Could you check a few things on this model? Use its own coordinates, in mm. Face numbers are marked on the shaded views. A direction names the side the tool comes from. Give positions to 0.01 mm unless a question says otherwise; leave off trailing zeros. Loops run counter-clockwise (first coordinate to the right, second up) from the corner with the lowest first, then second, coordinate; pieces in that order, holes last. Notation, with made-up numbers: (77.5, 75) - (133.5, 75) arc R16 cw to (133.5, 87) - close; hole circle Ø5 at (-39.5, 11.5). An arc over 180 degrees is marked (long way). Write each question's results on one line, items separated by ' | '. Start each with the question number.
1) On a 3-axis mill with a long thin cutter (end or side, diameter ignored), from which of +Z, -Z, +X, -X, +Y, -Y can I reach the whole of each face in a straight line? I mean the marked faces 1 and 2. Say none if no direction works.
2) I want a section at C-C, the plane y = -28.5. Write out the boundary of the cut face in (x, z), and give its area (3 significant figures).
3) I want a section at D-D, the plane x = 10. Write out the boundary of the cut face in (y, z).
4) If I drill on probe 1 along X at (y, z) = (-1.2, -15); probe 2 along Z at (x, y) = (-21, -31), over which ranges is the centre line in solid material (lowest first)? Write a range as [from, to].
5) I want a section at A-A, the plane z = -15. Write out the boundary of the cut face in (x, y), and give its area (3 significant figures).
6) I want a section at B-B, the plane x = 0. Write out the boundary of the cut face in (y, z).
7) I'm going to push flat-ended pins straight in: pin 1 (5 mm diameter, centred on x = -9.9, y = -15.2, fed in from +Z); pin 2 (12 mm diameter, centred on x = 5, z = -18, fed in from -Y); pin 3 (5 mm diameter, centred on x = 9.9, y = -15.2, fed in from -Z). Where does each tip first touch, or does it pass through?
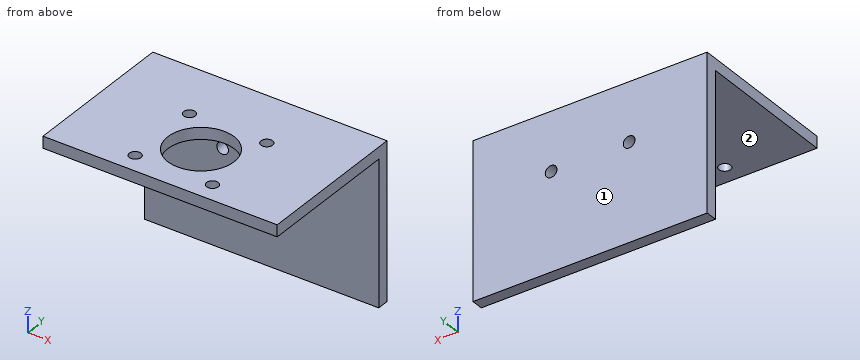
from build123d import *

# Parameters (mm, degrees)
BOSS_EXTRUDE1_DEPTH      = 30
BOSS_EXTRUDE1_DEPTH_BACK = 30
SKETCH2_R                = 1.5
SKETCH2_R_2              = 8.5
CUT_EXTRUDE1_DEPTH       = 30
SKETCH3_R                = 1.5
CUT_EXTRUDE2_DEPTH       = 30


with BuildPart() as part:
    # Sketch1 → Boss-Extrude1 (new, two sides: drawn at the far end of the back side and taken through both)
    with BuildSketch(Plane(origin=(0, 0, 0), x_dir=(0, 0, -1), z_dir=(1, 0, 0)).offset(-BOSS_EXTRUDE1_DEPTH_BACK)):
        Polygon((0, 0), (40, 0), (40, -3), (3, -3), (3, -40), (0, -40), align=None)
    extrude(amount=BOSS_EXTRUDE1_DEPTH + BOSS_EXTRUDE1_DEPTH_BACK)

    # Sketch2 → Cut-Extrude1 (cut)
    with BuildSketch(Plane.XY):
        with Locations((-9.8995, -15.201)):
            Circle(SKETCH2_R)
        with Locations((9.8995, -15.201)):
            Circle(SKETCH2_R)
        with Locations((-9.8995, -35)):
            Circle(SKETCH2_R)
        with Locations((9.8995, -35)):
            Circle(SKETCH2_R)
        with Locations((0, -25.101)):
            Circle(SKETCH2_R_2)
    extrude(amount=-CUT_EXTRUDE1_DEPTH, mode=Mode.SUBTRACT)

    # Sketch3 → Cut-Extrude2 (cut)
    with BuildSketch(Plane(origin=(0, 0, 0), x_dir=(1, 0, 0), z_dir=(0, 1, 0))):
        with Locations(Location((-10, 15, 0), (0, 0, 270))):
            Circle(SKETCH3_R)
        with Locations(Location((10, 15, 0), (0, 0, 270))):
            Circle(SKETCH3_R)
    extrude(amount=-CUT_EXTRUDE2_DEPTH, mode=Mode.SUBTRACT)


solid = part.part
Answers:
1) face 1: +Z, -Z, +X, -X, +Y | face 2: -Z, +X, -X, -Y
2) outline: (-30, -3) - (-7.79, -3) - (-7.79, 0) - (-30, 0) - close; (7.79, -3) - (30, -3) - (30, 0) - (7.79, 0) - close | area: 133 mm2
3) outline: (-40, -3) - (-36.5, -3) - (-36.5, 0) - (-40, 0) - close; (-33.5, -3) - (-16.7, -3) - (-16.7, 0) - (-33.5, 0) - close; (-13.7, -3) - (-3, -3) - (-3, -13.5) - (0, -13.5) - (0, 0) - (-13.7, 0) - close; (-3, -40) - (0, -40) - (0, -16.5) - (-3, -16.5) - close
4) probe 1: x = [-30, -11.5], [-8.5, 8.5], [11.5, 30] | probe 2: z = [-3, 0]
5) outline: (-30, -3) - (-11.5, -3) - (-11.5, 0) - (-30, 0) - close; (-8.5, -3) - (8.5, -3) - (8.5, 0) - (-8.5, 0) - close; (11.5, -3) - (30, -3) - (30, 0) - (11.5, 0) - close | area: 162 mm2
6) outline: (-40, -3) - (-33.6, -3) - (-33.6, 0) - (-40, 0) - close; (-16.6, -3) - (-3, -3) - (-3, -40) - (0, -40) - (0, 0) - (-16.6, 0) - close
7) pin 1: stops at z = 0 | pin 2: stops at y = -3 | pin 3: stops at z = -3
